```python
from build123d import *

# Parameters (mm, degrees)
BOSS_EXTRUDE1_DEPTH = 50
SKETCH2_R           = 2.5
CUT_EXTRUDE1_DEPTH  = 83.006097334
SKETCH3_R           = 1.5
CUT_EXTRUDE2_DEPTH  = 12.4
CHAMFER1_SIZE       = 2


with BuildPart() as part:
    # Sketch1 → Boss-Extrude1 (new, symmetric)
    with BuildSketch(Plane.XY):
        Polygon((-60, 0), (60, 0), (60, 20), (55, 25), (-47.875644347, 25), (-60, 4), align=None)
    extrude(amount=BOSS_EXTRUDE1_DEPTH, both=True)

    # Sketch2 → Cut-Extrude1 (cut, through all)
    with BuildSketch(Plane(origin=(0, 25, 0), x_dir=(1, 0, 0), z_dir=(0, 1, 0))):
        with Locations(Location((-32.5, 32.5, 0), (0, 0, 180))):
            Circle(SKETCH2_R)
        with Locations((-32.5, -32.5)):
            Circle(SKETCH2_R)
    cut_extrude1 = extrude(amount=-CUT_EXTRUDE1_DEPTH, mode=Mode.SUBTRACT)

    # Mirror1: Cut-Extrude1 across plane
    add(cut_extrude1.mirror(Plane(origin=(0, 0, 0), x_dir=(0, 0, 1), z_dir=(1, 0, 0))), mode=Mode.SUBTRACT)

    # Sketch3 → Cut-Extrude2 (cut)
    with BuildSketch(Plane(origin=(-46.732050808, 26.980762114, 0), x_dir=(0, 0, 1), z_dir=(-0.8660254037844384, 0.5000000000000007, 0))):
        with Locations(Location((-25, -14.411542732, 0), (0, 0, 270))):
            Circle(SKETCH3_R)
        with Locations(Location((27, -14.411542732, 0), (0, 0, 270))):
            Circle(SKETCH3_R)
    extrude(amount=-CUT_EXTRUDE2_DEPTH, mode=Mode.SUBTRACT)

    # Chamfer1
    chamfer1_edges = [part.edges().sort_by_distance(p)[0] for p in [
        (3.562177826, 25, 50),
        (3.562177826, 25, -50),
    ]]
    chamfer(chamfer1_edges, length=CHAMFER1_SIZE)


solid = part.part
```
Build history of the part. All positions in model axes, mm. A direction names the side the tool comes from. Coordinates: 2 decimals unless noted, no trailing zeros. Order: outer loops, then holes, each group sorted by start corner. A loop starts at its lowest first (then second) coordinate and runs counter-clockwise, first axis right, second up. Notation, with made-up numbers: M 4.5,-12.75 L 30.5,-12.75 A19 cw 30.5,19.25 Z; hole C -4.75,52 d4. An arc over 180 degrees is marked long. One line per question, with ' | ' between items. Start each with the question number.
1. Flat gauge pins, fed straight in: P1, Ø3, axis at x = -32.5, z = 32.5, coming from the +Y side; P2, Ø4, axis at y = 12.5, z = -9, coming from the -X side. Where does each tip first touch, or does it go through?
2. Wall check: line 1 along X through (y, z) = (13.5, 32.5); line 2 along Y through (x, z) = (-49, 9.5); line 3 along Y through (x, z) = (-49.5, 32.5). Give the ranges that are in metal, low to high. Write a range as [from, to].
3. Cut at D-D (z = -41). Write the cut outline in (x, y), plus the area to 3 significant figures.
4. Tool access for faces 1 (the face through (-43.2, 8.3, -25)), 2 (the face through (-1, 12, 50)): list every direction of +Z, -Z, +X, -X, +Y, -Y with a clear straight run to the whole face (end or side of a thin tool).
5. Cut at C-C (y = 18.25). Write the cut outline in (x, z), plus the area to 3 significant figures.
6. Cut at B-B (z = 32.5). Write the cut outline in (x, y).
7. Mould opens along Y. For faces 3 (the face through (-43.2, 8.3, 27)), 4 (the face through (32.17, 12.68, -30.02)), 5 (the face through (-53.85, 14.65, 0.7)) say: +Y half, -Y half, draft (parallel to the pull), parting line (faces both ways), or undercut.
8. Cut at A-A (x = -32.5). Write the cut outline in (y, z).
The answers:
1) P1: passes through | P2: stops at x = -56.25
2) line 1: x = [-54.52, -35], [-30, 30], [35, 60] | line 2: y = [0, 23.05] | line 3: y = [0, 22.19]
3) outline: M -60,0 L 60,0 L 60,20 L 55,25 L -47.88,25 L -60,4 Z | area: 2,860 mm2
4) face 1: none | face 2: +Z, +X, -X, +Y, -Y
5) outline: M -51.77,-50 L 60,-50 L 60,50 L -51.77,50 Z; hole C -32.5,-32.5 d5; hole C -32.5,32.5 d5; hole C 32.5,-32.5 d5; hole C 32.5,32.5 d5 | area: 11,100 mm2
6) outline: M -60,0 L -35,0 L -35,25 L -47.88,25 L -60,4 Z; M -30,0 L 30,0 L 30,25 L -30,25 Z; M 35,0 L 60,0 L 60,20 L 55,25 L 35,25 Z
7) face 3: undercut | face 4: draft | face 5: +Y half
8) outline: M 0,-50 L 23,-50 L 25,-48 L 25,-35 L 0,-35 Z; M 0,-30 L 25,-30 L 25,30 L 0,30 Z; M 0,35 L 25,35 L 25,48 L 23,50 L 0,50 Z
